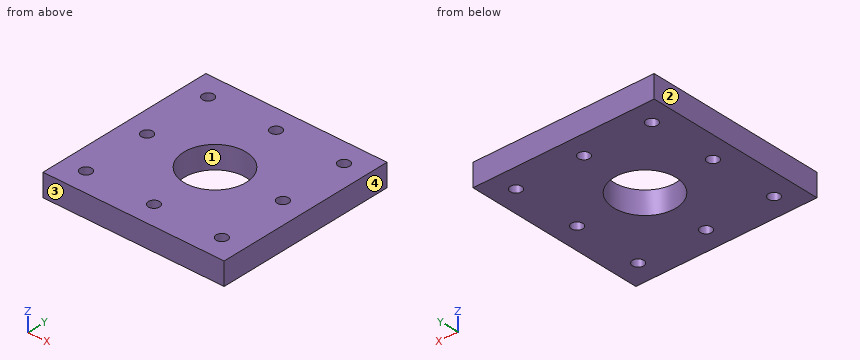
from build123d import *

# Parameters (mm, degrees)
SKETCH1_W           = 50.8
SKETCH1_H           = 50.8
BOSS_EXTRUDE1_DEPTH = 6.35
SKETCH2_R           = 8.73125
CUT_EXTRUDE7_DEPTH  = 7.35
SKETCH5_R           = 1.5875
CUT_EXTRUDE8_DEPTH  = 7.35
SKETCH7_R           = 1.5875
CUT_EXTRUDE9_DEPTH  = 7.35


with BuildPart() as part:
    # Sketch1 → Boss-Extrude1 (new body)
    with BuildSketch(Plane.XY):
        with Locations((25.4, 25.4)):
            Rectangle(SKETCH1_W, SKETCH1_H)
    extrude(amount=BOSS_EXTRUDE1_DEPTH)

    # Sketch2 → Cut-Extrude7 (cut, through all)
    with BuildSketch(Plane(origin=(0, 0, 0), x_dir=(-1, 0, 0), z_dir=(0, 0, -1))):
        with Locations((-25.4, 25.4)):
            Circle(SKETCH2_R)
    extrude(amount=-CUT_EXTRUDE7_DEPTH, mode=Mode.SUBTRACT)

    # Sketch5 → Cut-Extrude8 (cut, through all)
    with BuildSketch(Plane.XY.offset(6.35)):
        with Locations((25.4, 6.35)):
            Circle(SKETCH5_R)
        with Locations((6.35, 25.4)):
            Circle(SKETCH5_R)
        with Locations((25.4, 44.45)):
            Circle(SKETCH5_R)
        with Locations((44.45, 25.4)):
            Circle(SKETCH5_R)
    extrude(amount=-CUT_EXTRUDE8_DEPTH, mode=Mode.SUBTRACT)

    # Sketch7 → Cut-Extrude9 (cut, through all)
    with BuildSketch(Plane(origin=(0, 0, 0), x_dir=(-1, 0, 0), z_dir=(0, 0, -1))):
        with Locations((-6.35, 6.35)):
            Circle(SKETCH7_R)
        with Locations((-44.45, 6.35)):
            Circle(SKETCH7_R)
        with Locations((-44.45, 44.45)):
            Circle(SKETCH7_R)
        with Locations((-6.35, 44.45)):
            Circle(SKETCH7_R)
    extrude(amount=-CUT_EXTRUDE9_DEPTH, mode=Mode.SUBTRACT)


solid = part.part
Read the model definition and answer for the solid it produces. Units are mm, in the model's axes. Face numbers are marked on the shaded views. Round coordinates to 2 decimals unless told otherwise and drop trailing zeros. Write each loop counter-clockwise with the first axis right and the second up, starting at its lowest first coordinate (ties: lowest second). Pieces come first, ordered by that corner, then holes.
Q1. The mould has two halves that part along X. Classify the marked faces 1, 2, 3 and 4: released by +X, released by -X, zero draft, split by the parting line, or undercut.
Values:
face 1: undercut
face 2: released by -X
face 3: zero draft
face 4: released by +X
Q2. Find section B-B on z = 4.75. State how many separate pieces and enclosed holes the cut face has, and give its area (3 significant figures).
Values:
separate pieces: 1
enclosed holes: 9
area: 2,280 mm2
Q3. Find section A-A on y = 25.4. Determine the outline of the cut face in (x, z), and give its area (3 significant figures).
Values:
outline: (0, 0) - (4.76, 0) - (4.76, 6.35) - (0, 6.35) - close; (7.94, 0) - (16.67, 0) - (16.67, 6.35) - (7.94, 6.35) - close; (34.13, 0) - (42.86, 0) - (42.86, 6.35) - (34.13, 6.35) - close; (46.04, 0) - (50.8, 0) - (50.8, 6.35) - (46.04, 6.35) - close
area: 171 mm2
Q4. Straight lines are drawn through the part: line 1 (Y direction, x = 44.45, z = 1.75); line 2 (Y direction, x = 25.4, z = 5.25); line 3 (X direction, y = 6, z = 1). For each, find the intervals that lie inside material, in ascending order.
Values:
line 1: y = 0 to 4.76, 7.94 to 23.81, 26.99 to 42.86, 46.04 to 50.8
line 2: y = 0 to 4.76, 7.94 to 16.67, 34.13 to 42.86, 46.04 to 50.8
line 3: x = 0 to 4.8, 7.9 to 23.85, 26.95 to 42.9, 46 to 50.8
Q5. Find section C-C on x = 44.45. Determine the outline of the cut face in (y, z).
Values:
outline: (0, 0) - (4.76, 0) - (4.76, 6.35) - (0, 6.35) - close; (7.94, 0) - (23.81, 0) - (23.81, 6.35) - (7.94, 6.35) - close; (26.99, 0) - (42.86, 0) - (42.86, 6.35) - (26.99, 6.35) - close; (46.04, 0) - (50.8, 0) - (50.8, 6.35) - (46.04, 6.35) - close
